Source: three-view drawing plus pictorial views. Frame: mm from the lowest corner of the part. Give positions to 0.01 mm unless a question says otherwise; leave off trailing zeros. Loops run counter-clockwise (first coordinate to the right, second up) from the corner with the lowest first, then second, coordinate; pieces in that order, holes last.
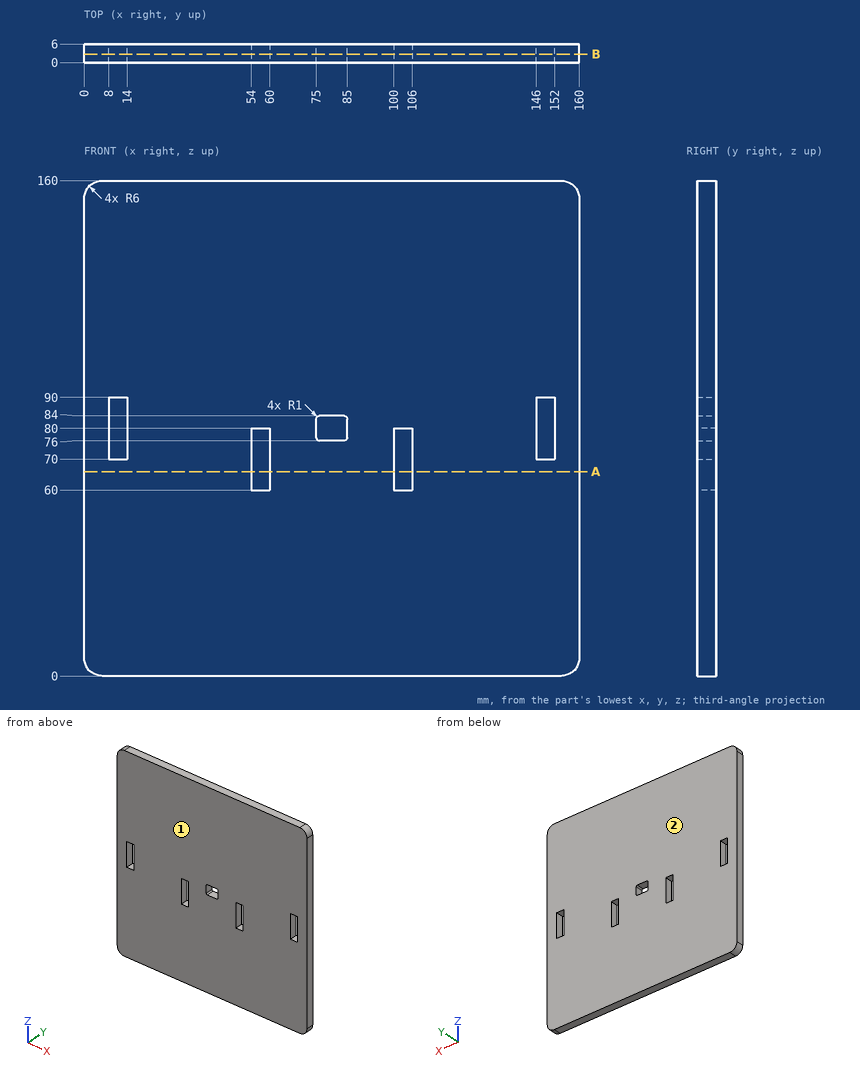
1) Ray query, probe 1 along X at (y, z) = (5.7, 62); probe 2 along X at (y, z) = (1.2, 80.5); probe 3 along X at (y, z) = (4.8, 77.5). Return the intervals inside material, ascending.
Checks:
probe 1: x = 0 to 54, 60 to 100, 106 to 160
probe 2: x = 0 to 8, 14 to 75, 85 to 146, 152 to 160
probe 3: x = 0 to 8, 14 to 54, 60 to 75, 85 to 100, 106 to 146, 152 to 160
2) Cut plane B-B (y = 2.75). State how many separate pieces and enclosed holes the cut face has, and give its area (3 significant figures).
Checks:
separate pieces: 1
enclosed holes: 5
area: 25,000 mm2
3) Cut plane A-A (z = 66). Return loops of the section in (x, y), and give its area (3 significant figures).
Checks:
outline: (0, 0) - (54, 0) - (54, 6) - (0, 6) - close; (60, 0) - (100, 0) - (100, 6) - (60, 6) - close; (106, 0) - (160, 0) - (160, 6) - (106, 6) - close
area: 888 mm2
4) Pull-direction query (Y, two-part tool) for the marked faces 1 and 2; classes: released by +Y, released by -Y, zero draft, split by the parting line, or undercut.
Checks:
face 1: released by -Y
face 2: released by +Y
